Geometry: final body of the model. Coordinates: model frame, mm. A direction names the side the tool comes from. Give positions to 0.01 mm unless a question says otherwise; leave off trailing zeros. Order: outer loops, then holes, each group sorted by start corner. A loop starts at its lowest first (then second) coordinate and runs counter-clockwise, first axis right, second up. Notation, with made-up numbers: (-4, 69) - (10, 69) arc R13 ccw to (10, 94) - close; hole circle Ø6 at (49, 34.25). An arc over 180 degrees is marked (long way). Use one line per item in the form item = value.
Autodesk Inventor part; units mm, degrees
ref_plane "YZ Plane" through (0, 0, 0) normal (1, 0, 0) x (0, 1, 0)
ref_plane "XZ Plane" through (0, 0, 0) normal (0, 1, 0) x (-1, 0, 0)
ref_plane "XY Plane" through (0, 0, 0) normal (0, 0, 1) x (1, 0, 0)
sketch "Sketch1" plane through (0, 0, 0) normal (0, 0, 1) x (1, 0, 0)
  line L0 (0, 0) -> (1.5, 0)
  line L1 (1.5, 0) -> (1.5, 10.5)
  line L2 (1.5, 10.5) -> (3, 12)
  line L3 (3, 12) -> (0, 12)
  line L4 (0, 12) -> (0, 0)
  line L5 (0, -2.4) -> (0, 14.4)
  dimension "d2" = 1.5
  dimension "d3" = 12
  dimension "d6" = 0
  dimension "d7" = 0
  dimension "d8" = 45
  dimension "d9" = 3
revolve "Revolution1" add sketch "Sketch1" angle 360 about axis through (0, -10, 0) along (0, 1, 0)
sketch "Sketch2" plane through (0, 12, 0) normal (0, 1, 0) x (1, 0, 0)
  circle A0 centre (0, 0) radius 3
  line L0 (-0.5, 5.0208) -> (0.5, 5.0208)
  line L1 (0.5, 5.0208) -> (0.5, -4.425)
  line L2 (0.5, -4.425) -> (-0.5, -4.425)
  line L3 (-0.5, -4.425) -> (-0.5, 5.0208)
  dimension "d10" = 1
  dimension "d11" = 0.5
extrude "Extrusion1" cut sketch "Sketch2" against normal blind 1 contours L1 A0 L3 | A0 L3 L0 L1 | L1 L2 L3 A0
thread "Thread2"
chamfer "Chamfer1" distance 0.2 angle 45 1 edges at (-1.5, 0, 0)
equation "\"d11\" = 0.5 * d10"
properties part number "XGEN_M3_screw"
(1) Contact query for flat-ended pins moving along their axis: pin 1 Ø0.5 at (x, z) = (0, 1) entering from +Y; pin 2 Ø3 at (x, y) = (0.5, 8) entering from +Z; pin 3 Ø2 at (x, z) = (2.5, 1) entering from -Y. Output: stop coordinate, or through.
Computed values:
pin_1 = 11
pin_2 = 1.5
pin_3 = 10.69
(2) Reachability of faces 1 (the face through (1, 12, 0)), 2 (the face through (-1.5, 5.42, -0.07)), 3 (the face through (-0.5, 11.5, 0)) from +Z, -Z, +X, -X, +Y, -Y: full face, straight path, thin tool, end or side. Return the list, or none.
Computed values:
face_1 = +Z, -Z, +X, -X, +Y
face_2 = -Y
face_3 = +Z, -Z, +Y
(3) Cut plane C-C on y = 11.25. Output: boundary loops of the cut face in (x, z).
Computed values:
outline = (-0.5, -2.19) - (-0.5, 2.19) arc R2.25 ccw to start; (0.5, -2.19) arc R2.25 ccw to (0.5, 2.19) - close
(4) Cut plane B-B on x = 0. Output: boundary loops of the cut face in (y, z).
Computed values:
outline = (0, -1.3) - (0.2, -1.5) - (10.5, -1.5) - (11, -2) - (11, 2) - (10.5, 1.5) - (0.2, 1.5) - (0, 1.3) - close
(5) Ray query, line 1 along X through (y, z) = (9.75, 0); line 2 along X through (y, z) = (7.5, -0.9); line 3 along Y through (x, z) = (0.1, 1). Return the intervals inside material, ascending.
Computed values:
line_1 = -1.5 to 1.5
line_2 = -1.2 to 1.2
line_3 = 0 to 11
(6) Cut plane A-A on z = 0. Output: boundary loops of the cut face in (x, y), plus the area to 3 significant figures.
Computed values:
outline = (-3, 12) - (-1.5, 10.5) - (-1.5, 0.2) - (-1.3, 0) - (1.3, 0) - (1.5, 0.2) - (1.5, 10.5) - (3, 12) - (0.5, 12) - (0.5, 11) - (-0.5, 11) - (-0.5, 12) - close
area = 37.2 mm²
(7) Cut plane D-D on y = 3. Output: boundary loops of the cut face in (x, z).
Computed values:
outline = circle Ø3 at (0, 0)
